Verification items for the finished model (mm, model axes). Give positions to 0.01 mm unless a question says otherwise; leave off trailing zeros. Order: outer loops, then holes, each group sorted by start corner. A loop starts at its lowest first (then second) coordinate and runs counter-clockwise, first axis right, second up. Notation, with made-up numbers: (50, 19) - (91, 19) arc R15 ccw to (91, 43) - close; hole circle Ø6 at (50, 55). An arc over 180 degrees is marked (long way). Answer as a JSON object with one key per item and string values.
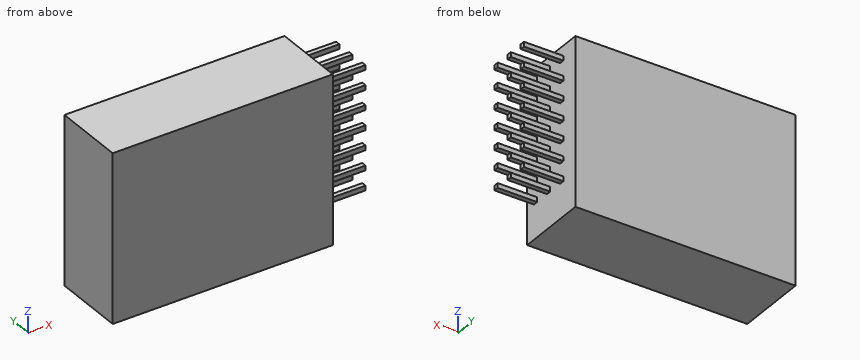
```python
from build123d import *

# Parameters (mm, degrees)
SKETCH1_W           = 28.3464
SKETCH1_H           = 21.59
BOSS_EXTRUDE1_DEPTH = 9.2456
SKETCH2_W           = 0.6096
SKETCH2_H           = 0.6096
BOSS_EXTRUDE2_DEPTH = 5.08
LPATTERN1_COUNT     = 7
LPATTERN1_PITCH     = 2.54


with BuildPart() as part:
    # Sketch1 → Boss-Extrude1 (new body)
    with BuildSketch(Plane(origin=(0, 0, 0), x_dir=(1, 0, 0), z_dir=(0, 1, 0))):
        with Locations((14.1732, 10.795)):
            Rectangle(SKETCH1_W, SKETCH1_H)
    extrude(amount=BOSS_EXTRUDE1_DEPTH)

    # Sketch2 → Boss-Extrude2 (add)
    with BuildSketch(Plane(origin=(28.3464, 0, 0), x_dir=(0, 0, -1), z_dir=(1, 0, 0))):
        with Locations((1.6002, 6.6294)):
            Rectangle(SKETCH2_W, SKETCH2_H)
        with Locations((1.6002, 1.6002)):
            Rectangle(SKETCH2_W, SKETCH2_H)
        with Locations((1.6002, 4.1148)):
            Rectangle(SKETCH2_W, SKETCH2_H)
    boss_extrude2 = extrude(amount=BOSS_EXTRUDE2_DEPTH)

    # LPattern1: Boss-Extrude2 ×7
    with Locations(*[(0, 0, -i * LPATTERN1_PITCH) for i in range(1, LPATTERN1_COUNT)]):
        add(boss_extrude2)


solid = part.part
```
(1) Material ranges on line 1 along X through (y, z) = (6.25, -3.5), recorded low to high. Write a range as [from, to].
Computed values:
{"line 1": "x = [0, 28.35]"}
(2) Section check B-B (z = -5). Record the cut outline in (x, y).
Computed values:
{"outline": "(0, 0) - (28.35, 0) - (28.35, 9.25) - (0, 9.25) - close"}
(3) Gauge pin test, flat ends, axial feed: pin 1 Ø0.7 at (x, y) = (30.5, 4) entering from -Z (3 decimals); pin 2 Ø0.5 at (x, y) = (29.5, 4) entering from +Z; pin 3 Ø0.7 at (x, z) = (30.5, -9.5) entering from +Y. Record the tip position at first contact, or that the pin passes through.
Computed values:
{"pin 1": "stops at z = -17.145", "pin 2": "stops at z = -1.3", "pin 3": "stops at y = 6.93"}
(4) Section check A-A (y = 5.25). Record the cut outline in (x, z).
Computed values:
{"outline": "(0, -21.59) - (28.35, -21.59) - (28.35, 0) - (0, 0) - close"}
